```python
from build123d import *

# Parameters (mm, degrees)
SKETCH1_R               = 2
BOSS_EXTRUDE1_DEPTH     = 4
BOSS_EXTRUDE2_START     = 4
BOSS_EXTRUDE2_DEPTH     = 9
CHAMFER2_SIZE           = 1
CHAMFER3_SIZE           = 1
CUT_EXTRUDE2_DEPTH      = 10
CUT_EXTRUDE2_DEPTH_BACK = 9
SKETCH1_2_R             = 2
SKETCH6_R               = 2
CUT_EXTRUDE3_DEPTH      = 17


with BuildPart() as part:
    # Sketch1 → Boss-Extrude1 (new body)
    with BuildSketch(Plane(origin=(0, 0, 0), x_dir=(1, 0, 0), z_dir=(0, 1, 0))):
        Polygon((-5, -2.310289343), (5, -2.310289343), (15, -0.310289343), (15, 5.689710657), (5, 7.689710657), (-5, 7.689710657), (-15, 5.689710657), (-15, -0.310289343), align=None)
        with Locations(Location((10, 2.689710657, 0), (0, 0, 270))):
            Circle(SKETCH1_R, mode=Mode.SUBTRACT)
        with Locations(Location((0, 2.689710657, 0), (0, 0, 270))):
            Circle(SKETCH1_R, mode=Mode.SUBTRACT)
        with Locations(Location((-10, 2.689710657, 0), (0, 0, 90))):
            Circle(SKETCH1_R, mode=Mode.SUBTRACT)
    boss_extrude1 = extrude(amount=BOSS_EXTRUDE1_DEPTH)

    # Sketch2 → Boss-Extrude2 (add)
    with BuildSketch(Plane(origin=(0, 0, 0), x_dir=(1, 0, 0), z_dir=(0, 1, 0)).offset(BOSS_EXTRUDE2_START)):
        Polygon((0, -2.310289343), (3.535533906, -0.845823249), (5, 2.689710657), (3.535533906, 6.225244563), (0, 7.689710657), (-3.535533906, 6.225244563), (-5, 2.689710657), (-3.535533906, -0.845823249), align=None)
    extrude(amount=BOSS_EXTRUDE2_DEPTH)

    # Mirror1: Boss-Extrude1 across plane
    add(boss_extrude1.mirror(Plane.ZX.offset(8.5)))

    # Chamfer2
    # the kernel refuses this chamfer: 1 mm, written as the material it takes off along each edge
    with BuildSketch(Plane(origin=(17.521742642, 4, -5.185362128), x_dir=(-0.19611613513818452, 0, 0.9805806756909201), z_dir=(-0.9805806756909201, 0, -0.19611613513818454))) as chamfer2_piece_1_section:
        Polygon((CHAMFER2_SIZE, 0), (0, -CHAMFER2_SIZE), (0, 0), align=None)
    chamfer2_piece_1 = extrude(amount=20.484770979, mode=Mode.PRIVATE)
    chamfer2_piece_1 = split(chamfer2_piece_1, bisect_by=Plane(origin=(15.841163755, 4, -1.128085786), z_dir=(0.38268343236508956, 0, -0.9238795325112868)), keep=Keep.TOP, mode=Mode.PRIVATE)
    add(chamfer2_piece_1, mode=Mode.SUBTRACT)
    with BuildSketch(Plane(origin=(15, 4, 2.881972331), x_dir=(-1, 0, 0), z_dir=(0, 0, -1))) as chamfer2_piece_2:
        Polygon((CHAMFER2_SIZE, 0), (0, -CHAMFER2_SIZE), (0, 0), align=None)
    extrude(amount=11.143365976, mode=Mode.SUBTRACT)
    with BuildSketch(Plane(origin=(-2.565227926, 4, 3.823334929), x_dir=(0, -1, 0), z_dir=(0.9805806756909202, 0, -0.19611613513818407))) as chamfer2_piece_3_section:
        Polygon((CHAMFER2_SIZE, 0), (0, CHAMFER2_SIZE), (0, 0), align=None)
    chamfer2_piece_3 = extrude(amount=20.484770979, mode=Mode.PRIVATE)
    chamfer2_piece_3 = split(chamfer2_piece_3, bisect_by=Plane(origin=(-2.724501391, 4, 3.43881477), z_dir=(0.38268343236508995, 0, 0.9238795325112867)), keep=Keep.TOP, mode=Mode.PRIVATE)
    add(chamfer2_piece_3, mode=Mode.SUBTRACT)
    with BuildSketch(Plane(origin=(10, 4, -2.689710657), x_dir=(0, 0, 1), z_dir=(-1, 0, 0))) as chamfer2_piece_4:
        Polygon((2 + CHAMFER2_SIZE, 0), (2, -CHAMFER2_SIZE), (2, 0), align=None)
    revolve(axis=Axis((10, 4, -2.689710657), (0, 1, 0)), mode=Mode.SUBTRACT)
    with BuildSketch(Plane(origin=(-2.565227926, 13, 3.823334929), x_dir=(-0.19611613513818407, 0, -0.9805806756909202), z_dir=(0.9805806756909202, 0, -0.19611613513818407))) as chamfer2_piece_5_section:
        Polygon((CHAMFER2_SIZE, 0), (0, CHAMFER2_SIZE), (0, 0), align=None)
    chamfer2_piece_5 = extrude(amount=20.484770979, mode=Mode.PRIVATE)
    chamfer2_piece_5 = split(chamfer2_piece_5, bisect_by=Plane(origin=(-2.724501391, 13, 3.43881477), z_dir=(0.38268343236508995, 0, 0.9238795325112867)), keep=Keep.TOP, mode=Mode.PRIVATE)
    add(chamfer2_piece_5, mode=Mode.SUBTRACT)
    with BuildSketch(Plane(origin=(17.521742642, 13, -5.185362128), x_dir=(-0.19611613513818452, 0, 0.9805806756909201), z_dir=(-0.9805806756909201, 0, -0.19611613513818454))) as chamfer2_piece_6_section:
        Polygon((CHAMFER2_SIZE, 0), (0, CHAMFER2_SIZE), (0, 0), align=None)
    chamfer2_piece_6 = extrude(amount=20.484770979, mode=Mode.PRIVATE)
    chamfer2_piece_6 = split(chamfer2_piece_6, bisect_by=Plane(origin=(15.841163755, 13, -1.128085786), z_dir=(0.38268343236508956, 0, -0.9238795325112868)), keep=Keep.TOP, mode=Mode.PRIVATE)
    add(chamfer2_piece_6, mode=Mode.SUBTRACT)
    with BuildSketch(Plane(origin=(15, 13, 2.881972331), x_dir=(-1, 0, 0), z_dir=(0, 0, -1))) as chamfer2_piece_7:
        Polygon((CHAMFER2_SIZE, 0), (0, CHAMFER2_SIZE), (0, 0), align=None)
    extrude(amount=11.143365976, mode=Mode.SUBTRACT)

    # Chamfer3
    # the kernel refuses this chamfer: 1 mm, written as the material it takes off along each edge
    with BuildSketch(Plane(origin=(-10, 4, -2.689710657), x_dir=(0, 0, -1), z_dir=(1, 0, 0))) as chamfer3_piece_1:
        Polygon((2 + CHAMFER3_SIZE, 0), (2, -CHAMFER3_SIZE), (2, 0), align=None)
    revolve(axis=Axis((-10, 4, -2.689710657), (0, 1, 0)), mode=Mode.SUBTRACT)
    with BuildSketch(Plane(origin=(2.565227926, 13, -9.202756242), x_dir=(0.19611613513818496, 0, 0.98058067569092), z_dir=(-0.98058067569092, 0, 0.19611613513818493))) as chamfer3_piece_2_section:
        Polygon((CHAMFER3_SIZE, 0), (0, CHAMFER3_SIZE), (0, 0), align=None)
    chamfer3_piece_2 = extrude(amount=20.484770979, mode=Mode.PRIVATE)
    chamfer3_piece_2 = split(chamfer3_piece_2, bisect_by=Plane(origin=(2.724501391, 13, -8.818236083), z_dir=(-0.38268343236509006, 0, -0.9238795325112867)), keep=Keep.TOP, mode=Mode.PRIVATE)
    add(chamfer3_piece_2, mode=Mode.SUBTRACT)
    with BuildSketch(Plane(origin=(-15, 13, -8.261393645), x_dir=(1, 0, 0), z_dir=(0, 0, 1))) as chamfer3_piece_3:
        Polygon((CHAMFER3_SIZE, 0), (0, CHAMFER3_SIZE), (0, 0), align=None)
    extrude(amount=11.143365976, mode=Mode.SUBTRACT)
    with BuildSketch(Plane(origin=(-17.521742642, 13, -0.194059185), x_dir=(0.19611613513818402, 0, -0.9805806756909202), z_dir=(0.9805806756909202, 0, 0.19611613513818402))) as chamfer3_piece_4_section:
        Polygon((CHAMFER3_SIZE, 0), (0, CHAMFER3_SIZE), (0, 0), align=None)
    chamfer3_piece_4 = extrude(amount=20.484770979, mode=Mode.PRIVATE)
    chamfer3_piece_4 = split(chamfer3_piece_4, bisect_by=Plane(origin=(-15.841163755, 13, -4.251335528), z_dir=(-0.3826834323650897, 0, 0.9238795325112868)), keep=Keep.TOP, mode=Mode.PRIVATE)
    add(chamfer3_piece_4, mode=Mode.SUBTRACT)
    with BuildSketch(Plane(origin=(2.565227926, 4, -9.202756242), x_dir=(0.19611613513818496, 0, 0.98058067569092), z_dir=(-0.98058067569092, 0, 0.19611613513818493))) as chamfer3_piece_5_section:
        Polygon((CHAMFER3_SIZE, 0), (0, -CHAMFER3_SIZE), (0, 0), align=None)
    chamfer3_piece_5 = extrude(amount=20.484770979, mode=Mode.PRIVATE)
    chamfer3_piece_5 = split(chamfer3_piece_5, bisect_by=Plane(origin=(2.724501391, 4, -8.818236083), z_dir=(-0.38268343236509006, 0, -0.9238795325112867)), keep=Keep.TOP, mode=Mode.PRIVATE)
    add(chamfer3_piece_5, mode=Mode.SUBTRACT)
    with BuildSketch(Plane(origin=(-15, 4, -8.261393645), x_dir=(1, 0, 0), z_dir=(0, 0, 1))) as chamfer3_piece_6:
        Polygon((CHAMFER3_SIZE, 0), (0, -CHAMFER3_SIZE), (0, 0), align=None)
    extrude(amount=11.143365976, mode=Mode.SUBTRACT)
    with BuildSketch(Plane(origin=(-17.521742642, 4, -0.194059185), x_dir=(0.19611613513818402, 0, -0.9805806756909202), z_dir=(0.9805806756909202, 0, 0.19611613513818402))) as chamfer3_piece_7_section:
        Polygon((CHAMFER3_SIZE, 0), (0, -CHAMFER3_SIZE), (0, 0), align=None)
    chamfer3_piece_7 = extrude(amount=20.484770979, mode=Mode.PRIVATE)
    chamfer3_piece_7 = split(chamfer3_piece_7, bisect_by=Plane(origin=(-15.841163755, 4, -4.251335528), z_dir=(-0.3826834323650897, 0, 0.9238795325112868)), keep=Keep.TOP, mode=Mode.PRIVATE)
    add(chamfer3_piece_7, mode=Mode.SUBTRACT)

    # Sketch1<2> → Cut-Extrude2 (cut, two sides: drawn at the far end of the back side and taken through both)
    with BuildSketch(Plane(origin=(0, 0, 0), x_dir=(1, 0, 0), z_dir=(0, 1, 0)).offset(-CUT_EXTRUDE2_DEPTH_BACK)):
        with Locations(Location((0, 2.689710657, 0), (0, 0, 270))):
            Circle(SKETCH1_2_R)
    extrude(amount=CUT_EXTRUDE2_DEPTH + CUT_EXTRUDE2_DEPTH_BACK, mode=Mode.SUBTRACT)

    # Sketch6 → Cut-Extrude3 (cut)
    with BuildSketch(Plane(origin=(0, 13, 0), x_dir=(1, 0, 0), z_dir=(0, 1, 0))):
        with Locations(Location((0, 2.689710657, 0), (0, 0, 270))):
            Circle(SKETCH6_R)
    extrude(amount=-CUT_EXTRUDE3_DEPTH, mode=Mode.SUBTRACT)


solid = part.part
```
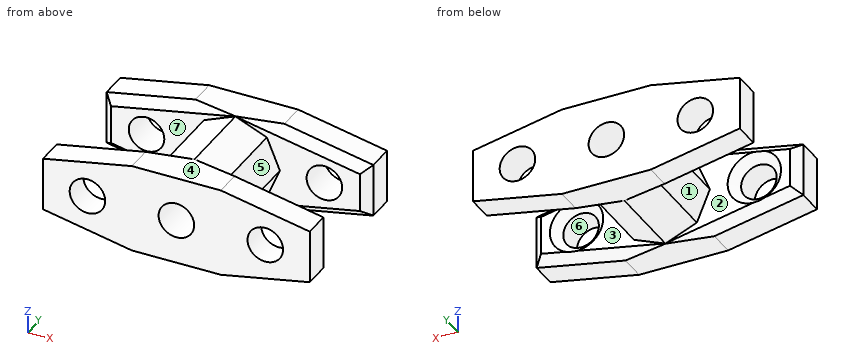
Here's how the part is built. I have some questions about the finished solid (model axes, mm). Face numbers are marked on the shaded views. A direction names the side the tool comes from. Give positions to 0.01 mm unless a question says otherwise; leave off trailing zeros. Order: outer loops, then holes, each group sorted by start corner. A loop starts at its lowest first (then second) coordinate and runs counter-clockwise, first axis right, second up. Notation, with made-up numbers: M -1.5,24 L 45.5,24 A11 ccw 45.5,34 Z; hole C 39.5,36 d1. An arc over 180 degrees is marked long. Use a Markdown table: item, result. Add a question column.
1. Suppose I cut it at C-C (z = -2). Give the number of separate pieces and of enclosed holes in the cut face, and give its area (3 significant figures).
2. Suppose I cut it at D-D (x = -4). List the corners of the cut face in (y, z) for me, and give its area (3 significant figures).
3. Suppose I cut it at A-A (y = 10.5). List the corners of the cut face in (x, z) for me.
4. Suppose I cut it at B-B (x = 5.5). List the corners of the cut face in (y, z) for me, and give its area (3 significant figures).
5. For pin 1 Ø1 at (y, z) = (10.5, -4) entering from +X; pin 2 Ø3.5 at (x, z) = (10, -2.69) entering from -Y; pin 3 Ø2 at (y, z) = (4.5, -2) entering from +X, each with a flat end and sliding along its axis, tell me the tip position at first contact or that it passes through.
6. If we mould it in two halves opening along Z, with no side actions, what happens to the marked faces 5, 6 and 7? For each: +Z half, -Z half, draft (parallel to the pull), parting line (faces both ways), or undercut.
7. On a 3-axis mill with a long thin cutter (end or side, diameter ignored), from which of +Z, -Z, +X, -X, +Y, -Y can I reach the whole of each face in a straight line? I mean the marked faces 1, 2, 3 and 4. Say none if no direction works.
8. I need wall thicknesses on probe 1 along Y at (x, z) = (-5, -6); probe 2 along X at (y, z) = (1.25, -4); probe 3 along X at (y, z) = (13.75, -4.5). Which ranges of each line are inside material? Lowest first, please. Write a range as from..to.
Results list:
| question | item | result |
|---|---|---|
| 1 | separate pieces | 6 |
| 1 | enclosed holes | 0 |
| 1 | area | 197 mm² |
| 2 | outline | M 0,-7.69 L 3.2,-7.69 L 4,-6.87 L 4,-5.1 L 13,-5.1 L 13,-6.87 L 13.8,-7.69 L 17,-7.69 L 17,2.31 L 13.8,2.31 L 13,1.49 L 13,-0.28 L 4,-0.28 L 4,1.49 L 3.2,2.31 L 0,2.31 Z |
| 2 | area | 122 mm² |
| 3 | outline | M -5,-2.69 L -3.54,-6.23 L 0,-7.69 L 3.54,-6.23 L 5,-2.69 L 3.54,0.85 L 0,2.31 L -3.54,0.85 Z; hole C 0,-2.69 d4 |
| 4 | outline | M 0,-7.59 L 3,-7.59 L 4,-6.57 L 4,1.19 L 3,2.21 L 0,2.21 Z; M 13,-6.57 L 14,-7.59 L 17,-7.59 L 17,2.21 L 14,2.21 L 13,1.19 Z |
| 4 | area | 76.4 mm² |
| 5 | pin 1 | stops at x = 4.66 |
| 5 | pin 2 | passes through |
| 5 | pin 3 | stops at x = 14.5 |
| 6 | face 5 | +Z half |
| 6 | face 6 | undercut |
| 6 | face 7 | draft |
| 7 | face 1 | -Z, -X |
| 7 | face 2 | -X |
| 7 | face 3 | +X |
| 7 | face 4 | +Z, +X, -X, +Y, -Y |
| 8 | probe 1 | y = 0..4, 13..17 |
| 8 | probe 2 | x = -15..-11.51, -8.49..-1.51, 1.51..8.49, 11.51..15 |
| 8 | probe 3 | x = -14.75..-10.85, -9.15..-0.85, 0.85..9.15, 10.85..14.75 |
